Here's how the part is built. I have some questions about the finished solid (model axes, mm). A direction names the side the tool comes from. Give positions to 0.01 mm unless a question says otherwise; leave off trailing zeros. Write each loop counter-clockwise with the first axis right and the second up, starting at its lowest first coordinate (ties: lowest second). Pieces come first, ordered by that corner, then holes. Notation, with made-up numbers: (54.25, -26.75) -> (86.25, -26.75) arc R34 ccw to (86.25, 4.25) -> close; hole circle Ø10 at (-28, 76). An arc over 180 degrees is marked (long way). Use one line per item in the form item = value.
```python
from build123d import *

# Parameters (mm, degrees)
BOSS_EXTRUDE1_DEPTH = 5
CUT_EXTRUDE1_DEPTH  = 3
SKETCH3_R           = 2.125
CUT_EXTRUDE2_DEPTH  = 0.5
SKETCH4_R           = 1
CUT_EXTRUDE3_DEPTH  = 5.5
BOSS_EXTRUDE2_DEPTH = 5
BOSS_EXTRUDE3_DEPTH = 15
SKETCH10_R          = 0.875
CUT_EXTRUDE6_DEPTH  = 6


with BuildPart() as part:
    # Sketch1 → Boss-Extrude1 (new body)
    with BuildSketch(Plane.XY):
        with BuildLine():
            Line((0, 5), (60, 5))
            ThreePointArc((60, 5), (65, 0), (60, -5))
            Line((60, -5), (0, -5))
            ThreePointArc((0, -5), (-5, 0), (0, 5))
        make_face()
    extrude(amount=BOSS_EXTRUDE1_DEPTH)

    # Sketch2 → Cut-Extrude1 (cut)
    with BuildSketch(Plane(origin=(0, 0, 0), x_dir=(-1, 0, 0), z_dir=(0, 0, -1))):
        with BuildLine():
            Line((2.344315233, -0.163358775), (2.25, 0))
            Line((2.25, 0), (2.344315233, 0.163358775))
            ThreePointArc((2.344315233, 0.163358775), (2.3210676, 0.367620993), (2.280056916, 0.56906982))
            Line((2.280056916, 0.56906982), (2.139877162, 0.695288237))
            Line((2.139877162, 0.695288237), (2.179095641, 0.879796675))
            ThreePointArc((2.179095641, 0.879796675), (2.093865332, 1.066877674), (1.992610742, 1.245793895))
            Line((1.992610742, 1.245793895), (1.820288237, 1.322516818))
            Line((1.820288237, 1.322516818), (1.800570985, 1.510113946))
            ThreePointArc((1.800570985, 1.510113946), (1.661700936, 1.661700936), (1.510113946, 1.800570985))
            Line((1.510113946, 1.800570985), (1.322516818, 1.820288237))
            Line((1.322516818, 1.820288237), (1.245793895, 1.992610742))
            ThreePointArc((1.245793895, 1.992610742), (1.066877674, 2.093865332), (0.879796675, 2.179095641))
            Line((0.879796675, 2.179095641), (0.695288237, 2.139877162))
            Line((0.695288237, 2.139877162), (0.56906982, 2.280056916))
            ThreePointArc((0.56906982, 2.280056916), (0.367620993, 2.3210676), (0.163358775, 2.344315233))
            Line((0.163358775, 2.344315233), (0, 2.25))
            Line((0, 2.25), (-0.163358775, 2.344315233))
            ThreePointArc((-0.163358775, 2.344315233), (-0.367620993, 2.3210676), (-0.56906982, 2.280056916))
            Line((-0.56906982, 2.280056916), (-0.695288237, 2.139877162))
            Line((-0.695288237, 2.139877162), (-0.879796675, 2.179095641))
            ThreePointArc((-0.879796675, 2.179095641), (-1.066877674, 2.093865332), (-1.245793895, 1.992610742))
            Line((-1.245793895, 1.992610742), (-1.322516818, 1.820288237))
            Line((-1.322516818, 1.820288237), (-1.510113946, 1.800570985))
            ThreePointArc((-1.510113946, 1.800570985), (-1.661700936, 1.661700936), (-1.800570985, 1.510113946))
            Line((-1.800570985, 1.510113946), (-1.820288237, 1.322516818))
            Line((-1.820288237, 1.322516818), (-1.992610742, 1.245793895))
            ThreePointArc((-1.992610742, 1.245793895), (-2.093865332, 1.066877674), (-2.179095641, 0.879796675))
            Line((-2.179095641, 0.879796675), (-2.139877162, 0.695288237))
            Line((-2.139877162, 0.695288237), (-2.280056916, 0.56906982))
            ThreePointArc((-2.280056916, 0.56906982), (-2.3210676, 0.367620993), (-2.344315233, 0.163358775))
            Line((-2.344315233, 0.163358775), (-2.25, 0))
            Line((-2.25, 0), (-2.344315233, -0.163358775))
            ThreePointArc((-2.344315233, -0.163358775), (-2.3210676, -0.367620993), (-2.280056916, -0.56906982))
            Line((-2.280056916, -0.56906982), (-2.139877162, -0.695288237))
            Line((-2.139877162, -0.695288237), (-2.179095641, -0.879796675))
            ThreePointArc((-2.179095641, -0.879796675), (-2.093865332, -1.066877674), (-1.992610742, -1.245793895))
            Line((-1.992610742, -1.245793895), (-1.820288237, -1.322516818))
            Line((-1.820288237, -1.322516818), (-1.800570985, -1.510113946))
            ThreePointArc((-1.800570985, -1.510113946), (-1.661700936, -1.661700936), (-1.510113946, -1.800570985))
            Line((-1.510113946, -1.800570985), (-1.322516818, -1.820288237))
            Line((-1.322516818, -1.820288237), (-1.245793895, -1.992610742))
            ThreePointArc((-1.245793895, -1.992610742), (-1.066877674, -2.093865332), (-0.879796675, -2.179095641))
            Line((-0.879796675, -2.179095641), (-0.695288237, -2.139877162))
            Line((-0.695288237, -2.139877162), (-0.56906982, -2.280056916))
            ThreePointArc((-0.56906982, -2.280056916), (-0.367620993, -2.3210676), (-0.163358775, -2.344315233))
            Line((-0.163358775, -2.344315233), (0, -2.25))
            Line((0, -2.25), (0.163358775, -2.344315233))
            ThreePointArc((0.163358775, -2.344315233), (0.367620993, -2.3210676), (0.56906982, -2.280056916))
            Line((0.56906982, -2.280056916), (0.695288237, -2.139877162))
            Line((0.695288237, -2.139877162), (0.879796675, -2.179095641))
            ThreePointArc((0.879796675, -2.179095641), (1.066877674, -2.093865332), (1.245793895, -1.992610742))
            Line((1.245793895, -1.992610742), (1.322516818, -1.820288237))
            Line((1.322516818, -1.820288237), (1.510113946, -1.800570985))
            ThreePointArc((1.510113946, -1.800570985), (1.661700936, -1.661700936), (1.800570985, -1.510113946))
            Line((1.800570985, -1.510113946), (1.820288237, -1.322516818))
            Line((1.820288237, -1.322516818), (1.992610742, -1.245793895))
            ThreePointArc((1.992610742, -1.245793895), (2.093865332, -1.066877674), (2.179095641, -0.879796675))
            Line((2.179095641, -0.879796675), (2.139877162, -0.695288237))
            Line((2.139877162, -0.695288237), (2.280056916, -0.56906982))
            ThreePointArc((2.280056916, -0.56906982), (2.3210676, -0.367620993), (2.344315233, -0.163358775))
        make_face()
    extrude(amount=-CUT_EXTRUDE1_DEPTH, mode=Mode.SUBTRACT)

    # Sketch3 → Cut-Extrude2 (cut)
    with BuildSketch(Plane.XY.offset(5)):
        Circle(SKETCH3_R)
    extrude(amount=-CUT_EXTRUDE2_DEPTH, mode=Mode.SUBTRACT)

    # Sketch4 → Cut-Extrude3 (cut, through all)
    with BuildSketch(Plane.XY.offset(4.5)):
        Circle(SKETCH4_R)
    extrude(amount=-CUT_EXTRUDE3_DEPTH, mode=Mode.SUBTRACT)

    # Sketch5 → Boss-Extrude2 (add)
    with BuildSketch(Plane(origin=(0, 0, 0), x_dir=(-1, 0, 0), z_dir=(0, 0, -1))):
        with BuildLine():
            Line((-60, 5), (-37.85, 5))
            Line((-37.85, 5), (-37.85, 7.75))
            Line((-37.85, 7.75), (-57.25, 7.75))
            ThreePointArc((-57.25, 7.75), (-62.730077554, 5.480077554), (-65, 0))
            ThreePointArc((-65, 0), (-63.535533906, 3.535533906), (-60, 5))
        make_face()
        with BuildLine():
            ThreePointArc((-60, -5), (-63.535533906, -3.535533906), (-65, 0))
            ThreePointArc((-65, 0), (-62.730077554, -5.480077554), (-57.25, -7.75))
            Line((-57.25, -7.75), (-37.85, -7.75))
            Line((-37.85, -7.75), (-37.85, -5))
            Line((-37.85, -5), (-60, -5))
        make_face()
    extrude(amount=-BOSS_EXTRUDE2_DEPTH)

    # Sketch6 → Boss-Extrude3 (add)
    with BuildSketch(Plane(origin=(0, 0, 0), x_dir=(-1, 0, 0), z_dir=(0, 0, -1))):
        with BuildLine():
            Line((-62.333306011, -5.85), (-41.85, -5.85))
            Line((-41.85, -5.85), (-41.85, 5.85))
            Line((-41.85, 5.85), (-62.333306011, 5.85))
            ThreePointArc((-62.333306011, 5.85), (-59.96339271, 7.259476565), (-57.25, 7.75))
            Line((-57.25, 7.75), (-37.85, 7.75))
            Line((-37.85, 7.75), (-37.85, 5))
            Line((-37.85, 5), (-37.85, -5))
            Line((-37.85, -5), (-37.85, -7.75))
            Line((-37.85, -7.75), (-57.25, -7.75))
            ThreePointArc((-57.25, -7.75), (-59.96339271, -7.259476565), (-62.333306011, -5.85))
        make_face()
    extrude(amount=BOSS_EXTRUDE3_DEPTH)

    # Sketch10 → Cut-Extrude6 (cut)
    with BuildSketch(Plane(origin=(0, 0, -15), x_dir=(-1, 0, 0), z_dir=(0, 0, -1))):
        with Locations((-39.9, 0)):
            Circle(SKETCH10_R)
    extrude(amount=-CUT_EXTRUDE6_DEPTH, mode=Mode.SUBTRACT)


solid = part.part
```
Q1. If I drill on line 1 along Y through (x, z) = (39.9, -11.7) (3 decimals); line 2 along Y through (x, z) = (0, 4.85) (3 decimals); line 3 along X through (y, z) = (1.25, -12.75), over which ranges is the centre line in solid material (lowest first)? Write a range as from..to.
Result set:
line_1 = -7.75..-0.875, 0.875..7.75
line_2 = -5..-2.125, 2.125..5
line_3 = 37.85..41.85
Q2. Which directions (+Z, -Z, +X, -X, +Y, -Y) give clear straight access to the entire face, cutting with the end or side of a thin tool? Please do faces 1 (the face through (19, -5, 2)), 2 (the face through (40, 0, -9)), 3 (the face through (19, 5, 2)), 4 (the face through (54, 0, 0)).
Result set:
face_1 = +Z, -Z, -X, -Y
face_2 = -Z
face_3 = +Z, -Z, -X, +Y
face_4 = -Z, +X
Q3. I want a section at C-C, the plane x = 54. Write out the boundary of the cut face in (y, z), and give its area (4 significant figures).
Result set:
outline = (-7.75, -15) -> (-5.85, -15) -> (-5.85, 0) -> (5.85, 0) -> (5.85, -15) -> (7.75, -15) -> (7.75, 5) -> (-7.75, 5) -> close
area = 134.5 mm2
Q4. Will these pins go through, and if not, where does the flat tip stop? pin 1 Ø4 at (x, y) = (1, 0) entering from -Z; pin 2 Ø1.5 at (x, z) = (16.5, 3.5) entering from +Y; pin 3 Ø2 at (y, z) = (-4, -10) entering from -X.
Result set:
pin_1 = 0
pin_2 = 5
pin_3 = 37.85
Q5. I want a section at D-D, the plane x = 32.5. Write out the boundary of the cut face in (y, z).
Result set:
outline = (-5, 0) -> (5, 0) -> (5, 5) -> (-5, 5) -> close
Q6. I want a section at A-A, the plane z = -11.5. Write out the boundary of the cut face in (x, y) (3 decimals).
Result set:
outline = (37.85, -7.75) -> (57.25, -7.75) arc R7.75 ccw to (62.333, -5.85) -> (41.85, -5.85) -> (41.85, 5.85) -> (62.333, 5.85) arc R7.75 ccw to (57.25, 7.75) -> (37.85, 7.75) -> close; hole circle Ø1.75 at (39.9, 0)
Q7. I want a section at B-B, the plane x = 39.9. Write out the boundary of the cut face in (y, z) (3 decimals), and give its area (4 significant figures).
Result set:
outline = (-7.75, -15) -> (-0.875, -15) -> (-0.875, -9) -> (0.875, -9) -> (0.875, -15) -> (7.75, -15) -> (7.75, 5) -> (-7.75, 5) -> close
area = 299.5 mm2
Q8. If we mould it in two halves opening along Y, with no side actions, what happens to faces 5 (the face through (48, 7.75, -5)), 6 (the face through (41.85, 0, -7)), 7 (the face through (37.85, 0, -5))? For each: +Y half, -Y half, draft (parallel to the pull), parting line (faces both ways), or undercut.
Result set:
face_5 = +Y half
face_6 = undercut
face_7 = draft
